```python
from build123d import *

# Parameters (mm, degrees)
F0_W     = 36.86
F0_H     = 30.5
F1_DEPTH = 6
F2_R     = 1.7
F3_DEPTH = 25
F4_W     = 8.913981
F4_H     = 1.5
F5_DEPTH = 26


with BuildPart() as f1:
    # F0 (on Top) → F1 (new body)
    with BuildSketch(Plane.XY):
        Rectangle(F0_W, F0_H)
    extrude(amount=F1_DEPTH)

    # F2 (on face) → F3 (cut)
    with BuildSketch(Plane.XY.offset(6)):
        with Locations((-11.43, 11.05)):
            Circle(F2_R)
        with Locations((11.43, 11.05)):
            Circle(F2_R)
    extrude(amount=-F3_DEPTH, mode=Mode.SUBTRACT)

    # F4 (on face) → F5 (join)
    with BuildSketch(Plane.XY.offset(6)):
        Polygon((-7.61, 6.7), (-7.61, -11.3), (-4.264409, -11.3), (4.649572, -11.3), (7.61, -11.3), (7.61, 6.7), align=None)
        with Locations((0.192582, -12.05)):
            Rectangle(F4_W, F4_H)
    extrude(amount=F5_DEPTH)


solid = f1.part
```
For this review, take the finished solid that the model builds, in its own axes (mm). A direction names the side the tool comes from. Round coordinates to 2 decimals unless told otherwise and drop trailing zeros. Write each loop counter-clockwise with the first axis right and the second up, starting at its lowest first coordinate (ties: lowest second). Pieces come first, ordered by that corner, then holes. Notation, with made-up numbers: (77, 50.5) - (136, 50.5) arc R19 ccw to (136, 75.5) - close; hole circle Ø1 at (21.25, 5.25). An arc over 180 degrees is marked (long way). Write each question's results on one line, items separated by ' | '.
Item 1: To check wall thickness, follow line 1 along X through (y, z) = (11, 5); line 2 along Y through (x, z) = (-11.43, 3.1); line 3 along X through (y, z) = (-4, 26). State the ranges of each line that lie inside material, in increasing order. Write a range as from..to.
Calculated:
line 1: x = -18.43..-13.13, -9.73..9.73, 13.13..18.43 | line 2: y = -15.25..9.35, 12.75..15.25 | line 3: x = -7.61..7.61
Item 2: Take a section at B-B on z = 2. State the section outline as (x, y) points, then the cut area to 3 significant figures.
Calculated:
outline: (-18.43, -15.25) - (18.43, -15.25) - (18.43, 15.25) - (-18.43, 15.25) - close; hole circle Ø3.4 at (-11.43, 11.05); hole circle Ø3.4 at (11.43, 11.05) | area: 1,110 mm^2
Item 3: For pin 1 (12 mm diameter, centred on x = -8.5, z = 17, fed in from -Y); pin 2 (12 mm diameter, centred on x = -1, z = 20.5, fed in from +Y); pin 3 (14.5 mm diameter, centred on y = -5, z = 21.5, fed in from -X); pin 4 (4 mm diameter, centred on x = -11.43, y = 11.05, fed in from -Z), all flat-tipped, find the tip position at first contact; note any pin that passes through.
Calculated:
pin 1: stops at y = -12.8 | pin 2: stops at y = 6.7 | pin 3: stops at x = -7.61 | pin 4: stops at z = 0
Item 4: Draft analysis for pull direction Y (two halves, no side actions). For faces 6 (the face through (0, -12.8, 19)), 7 (the face through (-13.13, 11.12, 3.04)), 8 (the face through (-4.264, -12, 19)), state which applies: pulls with the +Y half, pulls with the -Y half, needs draft (parallel to the pull), parting line crosses it, or undercut.
Calculated:
face 6: pulls with the -Y half | face 7: undercut | face 8: needs draft
Item 5: For faces 1 (the face through (7.61, -2, 19)), 2 (the face through (0, 6.7, 19)), 3 (the face through (-7.61, -2, 19)), 4 (the face through (6, -11.3, 19)), 5 (the face through (-6, -11.3, 19)), list the 3-axis set-ups (+Z, -Z, +X, -X, +Y, -Y) from which the entire face can be reached by the end or side of a thin tool; tool diameter is ignored.
Calculated:
face 1: +Z, +X, +Y, -Y | face 2: +Z, +X, -X, +Y | face 3: +Z, -X, +Y, -Y | face 4: +Z, +X, -Y | face 5: +Z, -X, -Y
Item 6: Take a section at D-D on y = 1. State the section outline as (x, z) points.
Calculated:
outline: (-18.43, 0) - (18.43, 0) - (18.43, 6) - (7.61, 6) - (7.61, 32) - (-7.61, 32) - (-7.61, 6) - (-18.43, 6) - close
Item 7: Take a section at A-A on y = 11.05. State the section outline as (x, z) points, then the cut area to 3 significant figures.
Calculated:
outline: (-18.43, 0) - (-13.13, 0) - (-13.13, 6) - (-18.43, 6) - close; (-9.73, 0) - (9.73, 0) - (9.73, 6) - (-9.73, 6) - close; (13.13, 0) - (18.43, 0) - (18.43, 6) - (13.13, 6) - close | area: 180 mm^2
Item 8: Take a section at C-C on x = -11.43. State the section outline as (y, z) points.
Calculated:
outline: (-15.25, 0) - (9.35, 0) - (9.35, 6) - (-15.25, 6) - close; (12.75, 0) - (15.25, 0) - (15.25, 6) - (12.75, 6) - close
